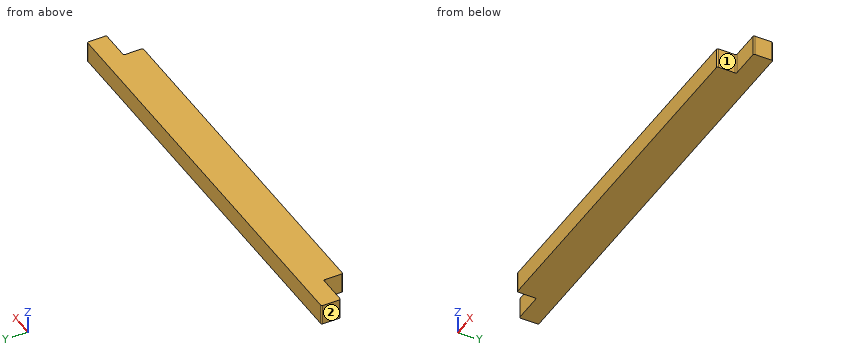
from build123d import *

# Parameters (mm, degrees)
SKETCH1_W           = 66.16
SKETCH1_H           = 6
BOSS_EXTRUDE1_DEPTH = 3.175
SKETCH2_W           = 4.85
SKETCH2_H           = 3
CUT_EXTRUDE1_DEPTH  = 34.367154883
FILLET1_R           = 0.2


with BuildPart() as part:
    # Sketch1 → Boss-Extrude1 (new body)
    with BuildSketch(Plane.XY):
        Rectangle(SKETCH1_W, SKETCH1_H)
    extrude(amount=BOSS_EXTRUDE1_DEPTH)

    # Sketch2 → Cut-Extrude1 (cut, through all)
    with BuildSketch(Plane.XY.offset(3.175)):
        with Locations((-30.655, -1.5)):
            Rectangle(SKETCH2_W, SKETCH2_H)
        with Locations((30.655, -1.5)):
            Rectangle(SKETCH2_W, SKETCH2_H)
    extrude(amount=-CUT_EXTRUDE1_DEPTH, mode=Mode.SUBTRACT)

    # Fillet1
    fillet1_edges = [part.edges().sort_by_distance(p)[0] for p in [
        (-33.08, 0, 1.5875),
        (-28.23, 0, 1.5875),
        (-28.23, -3, 1.5875),
        (33.08, 0, 1.5875),
        (28.23, -3, 1.5875),
        (28.23, 0, 1.5875),
        (-33.08, 3, 1.5875),
        (33.08, 3, 1.5875),
    ]]
    fillet(fillet1_edges, radius=FILLET1_R)


solid = part.part
The listing builds one solid part. Answer for the finished solid, in the listing's coordinates (mm). Face numbers are marked on the shaded views. A direction names the side the tool comes from. Round coordinates to 2 decimals unless told otherwise and drop trailing zeros. Loops run counter-clockwise (first coordinate to the right, second up) from the corner with the lowest first, then second, coordinate; pieces in that order, holes last. Notation, with made-up numbers: M 72,-27 L 98,-27 A15 ccw 98,-18 Z; hole C -33,-12 d1. An arc over 180 degrees is marked long. Write each question's results on one line, items separated by ' | '. Start each with the question number.
1) Find section A-A on z = 2.1. Write down the section's boundary in (x, y).
2) Which of the six approach directions +Z, -Z, +X, -X, +Y, -Y give full straight-line access (tool end or side, diameter ignored) to the marked faces 1 and 2?
3) Find section B-B on y = -0.8. Write down the section's boundary in (x, z) (3 decimals).
4) Each of these flat-tipped pins is pushed along its axis until it touches: pin 1 (1.6 mm diameter, centred on x = 30, z = 1.5, fed in from -Y); pin 2 (0.8 mm diameter, centred on y = -2, z = 1.5, fed in from -X). Where does it stop, or does it pass through?
5) A straight line is drawn through the part: probe 1 along X at (y, z) = (-0.7, 1.1). Find the intervals that lie inside material, in ascending order.
Final values:
1) outline: M -33.08,0.2 A0.2 ccw -32.88,0 L -28.43,0 A0.2 cw -28.23,-0.2 L -28.23,-2.8 A0.2 ccw -28.03,-3 L 28.03,-3 A0.2 ccw 28.23,-2.8 L 28.23,-0.2 A0.2 cw 28.43,0 L 32.88,0 A0.2 ccw 33.08,0.2 L 33.08,2.8 A0.2 ccw 32.88,3 L -32.88,3 A0.2 ccw -33.08,2.8 Z
2) face 1: +Z, -Z, +X, -Y | face 2: +Z, -Z, -X, +Y, -Y
3) outline: M -28.23,0 L 28.23,0 L 28.23,3.175 L -28.23,3.175 Z
4) pin 1: y = 0 | pin 2: x = -28.23
5) probe 1: -28.23 to 28.23
